Could you check a few things on this model? Use its own coordinates, in mm. Face numbers are marked on the shaded views. A direction names the side the tool comes from. Coordinates: 2 decimals unless noted, no trailing zeros. Order: outer loops, then holes, each group sorted by start corner. A loop starts at its lowest first (then second) coordinate and runs counter-clockwise, first axis right, second up. Notation, with made-up numbers: (63.5, 45.25) -> (96.5, 45.25) arc R29 ccw to (96.5, 71.25) -> close; hole circle Ø11 at (14.25, 66.5). An arc over 180 degrees is marked (long way). Put each result on its own line as item: value. Start each with the question number.
Q1. If we section it at A-A (z = -64): Please give me the cut outline in (x, y).
Q2. If we section it at B-B (x = 123.5): Please give me the cut outline in (y, z).
Q3. Please list where these lines run through material, in increasing order: line 1 along Z through (x, y) = (0, -72.5); line 2 along Z through (x, y) = (0, -67.75); line 3 along Z through (x, y) = (62.5, -3.5).
Q4. Will these pins go through, and if not, where does the flat tip stop? pin 1 (4 mm diameter, centred on y = -61.5, z = 25.5, fed in from +X); pin 2 (2 mm diameter, centred on x = 31, y = -31.5, fed in from +Z); pin 3 (6 mm diameter, centred on y = -16, z = -29.5, fed in from +X).
Q5. For the marked faces 5 and 6, which set-ups out of +Z, -Z, +X, -X, +Y, -Y let a thin tool reach every point of the face, with its end or its side?
Q6. We'd pull the mould along X, two halves only. Please class the marked faces 1, 2, 3 and 4: +X half, -X half, draft (parallel to the pull), parting line (faces both ways), or undercut.
from build123d import *

# Parameters (mm, degrees)
F0_R           = 19.05
F1_DEPTH       = 76.2
F3_D           = 38.1
F3_DEPTH       = 12.7
F3_CBORE_D     = 50.8
F3_CBORE_DEPTH = 6.35
F3_TIP         = 11.4463947925
F5_D           = 38.1
F5_DEPTH       = 12.7
F5_CBORE_D     = 50.8
F5_CBORE_DEPTH = 6.35
F5_TIP         = 11.4463947925


with BuildPart() as f1:
    # F0 (on Front) → F1 (new body)
    with BuildSketch(Plane.XZ):
        with BuildLine():
            ThreePointArc((-40.9769218572, 0), (0.2980781428, -41.275), (41.5730781428, 0))
            ThreePointArc((41.5730781428, 0), (0.2980781428, 41.275), (-40.9769218572, 0))
        make_face()
        with Locations((0.2980781428, 0)):
            Circle(F0_R, mode=Mode.SUBTRACT)
        with BuildLine():
            Line((41.5730781428, -45.8812290595), (41.5730781428, 0))
            ThreePointArc((41.5730781428, 0), (0.2980781428, -41.275), (-40.9769218572, 0))
            Line((-40.9769218572, 0), (-40.9769218572, -76.2))
            Line((-40.9769218572, -76.2), (136.8230781428, -76.2))
            Line((136.8230781428, -76.2), (136.2701599936, -45.8812290595))
            Line((136.2701599936, -45.8812290595), (41.5730781428, -45.8812290595))
        make_face()
        with Locations((0.2980781428, 0)):
            Circle(F0_R)
    extrude(amount=F1_DEPTH)

    # F3
    with Locations(Plane.XZ.offset(76.2)):
        with Locations((0, 0)):
            CounterBoreHole(F3_D / 2, F3_CBORE_D / 2, F3_CBORE_DEPTH, depth=F3_DEPTH)
            with Locations((0, 0, -(F3_DEPTH + F3_TIP / 2))):  # 118° drill point
                Cone(0, F3_D / 2, F3_TIP, mode=Mode.SUBTRACT)

    # F5
    with Locations(Plane.XY.offset(-45.8812290595)):
        with Locations((88.9216190682, -38.1)):
            CounterBoreHole(F5_D / 2, F5_CBORE_D / 2, F5_CBORE_DEPTH, depth=F5_DEPTH)
            with Locations((0, 0, -(F5_DEPTH + F5_TIP / 2))):  # 118° drill point
                Cone(0, F5_D / 2, F5_TIP, mode=Mode.SUBTRACT)


solid = f1.part
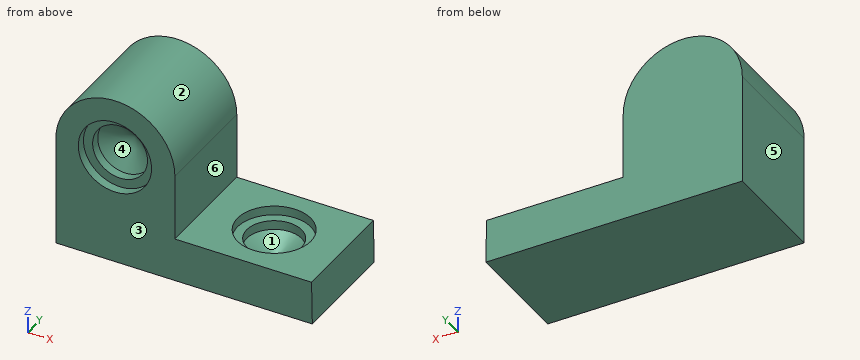
The answers:
1. outline: (-40.98, -76.2) -> (136.6, -76.2) -> (136.6, 0) -> (-40.98, 0) -> close; hole circle Ø20.06 at (88.92, -38.1)
2. outline: (-76.2, -76.2) -> (0, -76.2) -> (0, -45.88) -> (-76.2, -45.88) -> close
3. line 1: -76.2 to -25.4, 25.4 to 41.27
3. line 2: -76.2 to -19.05, 19.05 to 41.27
3. line 3: -76.2 to -45.88
4. pin 1: x = 34.23
4. pin 2: z = 28.66
4. pin 3: x = 41.57
5. face 5: +Z, -Z, -X, +Y, -Y
5. face 6: +Z, +X, +Y, -Y
6. face 1: undercut
6. face 2: parting line
6. face 3: draft
6. face 4: undercut
